from build123d import *

# Parameters (mm, degrees)
SKETCH2_R           = 8.5
SKETCH2_R_2         = 0.5
BOSS_EXTRUDE1_DEPTH = 20
SKETCH3_R           = 0.5
SKETCH3_R_2         = 2.3
CUT_EXTRUDE1_DEPTH  = 6
CUT_EXTRUDE2_DEPTH  = 12


with BuildPart() as part:
    # Sketch2 → Boss-Extrude1 (new body)
    with BuildSketch(Plane.XY):
        Circle(SKETCH2_R)
        with Locations((0, 1.5)):
            Circle(SKETCH2_R_2, mode=Mode.SUBTRACT)
    extrude(amount=BOSS_EXTRUDE1_DEPTH)

    # Sketch3 → Cut-Extrude1 (cut)
    with BuildSketch(Plane.XY):
        with Locations((0, 1.5)):
            Circle(SKETCH3_R)
        with Locations((-5, 1.5)):
            Circle(SKETCH3_R_2)
        with Locations((5, 1.5)):
            Circle(SKETCH3_R_2)
    extrude(amount=CUT_EXTRUDE1_DEPTH, mode=Mode.SUBTRACT)

    # Sketch5 → Cut-Extrude2 (cut)
    with BuildSketch(Plane.XY.offset(20)):
        with BuildLine():
            Line((-3.217141588, 4.2), (3.217141588, 4.2))
            ThreePointArc((3.217141588, 4.2), (0, -2.7), (-3.217141588, 4.2))
        make_face()
    extrude(amount=-CUT_EXTRUDE2_DEPTH, mode=Mode.SUBTRACT)


solid = part.part
Build history of the part. All positions in model axes, mm. A direction names the side the tool comes from. Round coordinates to 2 decimals unless told otherwise and drop trailing zeros. Loops run counter-clockwise (first coordinate to the right, second up) from the corner with the lowest first, then second, coordinate; pieces in that order, holes last. Notation, with made-up numbers: (85, 75.5) -> (93, 75.5) arc R26 ccw to (93, 100.5) -> close; hole circle Ø7 at (36, -8.75). An arc over 180 degrees is marked (long way). Use CSV: the item, a comma, the result in double quotes. Start each with the question number.
Q1. Mould opens along Y. For faces 1 (the face through (7.125, 0.619, 2.958)), 2 (the face through (4.57, 7.167, 9.86)), 3 (the face through (0, -4, 20)), 4 (the face through (-2.875, 0.619, 2.958)) say: +Y half, -Y half, draft (parallel to the pull), parting line (faces both ways), or undercut.
Q2. Drill centre lines: L1, parallel to Z at x = -4.75, y = 0; L2, parallel to Y at x = 4, z = 4.25; L3, parallel to Z at x = 2.25, y = -2. Where is each one in solid material? Low to high.
Q3. Saw through at D-D on x = -5.75. Give the cut face in (y, z), and give its area (3 significant figures).
Q4. Saw through at A-A on x = 0. Give the cut face in (y, z).
Q5. Saw through at B-B on y = 1.5. Give the cut face in (x, z).
Q6. Which spindle directions (+Z, -Z, +X, -X, +Y, -Y) get a long thin tool onto all of the face, cutting with end or side? Do faces 5 (the face through (0, 4.2, 14)), 6 (the face through (0, 2, 4)), 7 (the face through (-5, 2, 6)). Say none if no direction does.
Q7. Saw through at C-C on z = 15. Give the cut face in (x, y), and give its area (3 significant figures).
Q8. Flat gauge pins, fed straight in: pin 1 Ø4 at (x, z) = (-3, 13) entering from +Y; pin 2 Ø2 at (x, z) = (4.5, 7) entering from -Y; pin 3 Ø1 at (x, z) = (6.5, 11) entering from +Y; pin 4 Ø1.5 at (x, y) = (-5.5, 0) entering from -Z. Where does each tip first touch, or does it go through?
Solutions:
1,face 1,"undercut"
1,face 2,"parting line"
1,face 3,"draft"
1,face 4,"undercut"
2,L1,"z = 6 to 20"
2,L2,"y = -7.5 to -0.57, 3.57 to 7.5"
2,L3,"z = 0 to 8"
3,outline,"(-6.26, 0) -> (-0.67, 0) -> (-0.67, 6) -> (3.67, 6) -> (3.67, 0) -> (6.26, 0) -> (6.26, 20) -> (-6.26, 20) -> close"
3,area,"224 mm^2"
4,outline,"(-8.5, 0) -> (1, 0) -> (1, 8) -> (-2.7, 8) -> (-2.7, 20) -> (-8.5, 20) -> close; (2, 0) -> (8.5, 0) -> (8.5, 20) -> (4.2, 20) -> (4.2, 8) -> (2, 8) -> close"
5,outline,"(-8.37, 0) -> (-7.3, 0) -> (-7.3, 6) -> (-2.7, 6) -> (-2.7, 0) -> (-0.5, 0) -> (-0.5, 8) -> (-4.2, 8) -> (-4.2, 20) -> (-8.37, 20) -> close; (0.5, 0) -> (2.7, 0) -> (2.7, 6) -> (7.3, 6) -> (7.3, 0) -> (8.37, 0) -> (8.37, 20) -> (4.2, 20) -> (4.2, 8) -> (0.5, 8) -> close"
6,face 5,"+Z"
6,face 6,"+Z, -Z"
6,face 7,"-Z"
7,outline,"circle Ø17 at (0, 0); hole (-3.22, 4.2) arc R4.2 ccw (long way) to (3.22, 4.2) -> close"
7,area,"178 mm^2"
8,pin 1,"stops at y = 8.44"
8,pin 2,"stops at y = -7.75"
8,pin 3,"stops at y = 6.02"
8,pin 4,"stops at z = 0"
